Geometry check sheet. Reference: drawing and pictorial views, mm from the part's lowest x, y, z. A direction names the side the tool comes from. Coordinates: 2 decimals unless noted, no trailing zeros. Write each loop counter-clockwise with the first axis right and the second up, starting at its lowest first coordinate (ties: lowest second). Pieces come first, ordered by that corner, then holes. Notation, with made-up numbers: (52, 30.25) - (81, 30.25) arc R36 cw to (81, 69.25) - close; hole circle Ø4 at (3.5, 62). An arc over 180 degrees is marked (long way). Answer as a JSON object with one key per item and string values. Group by question number.
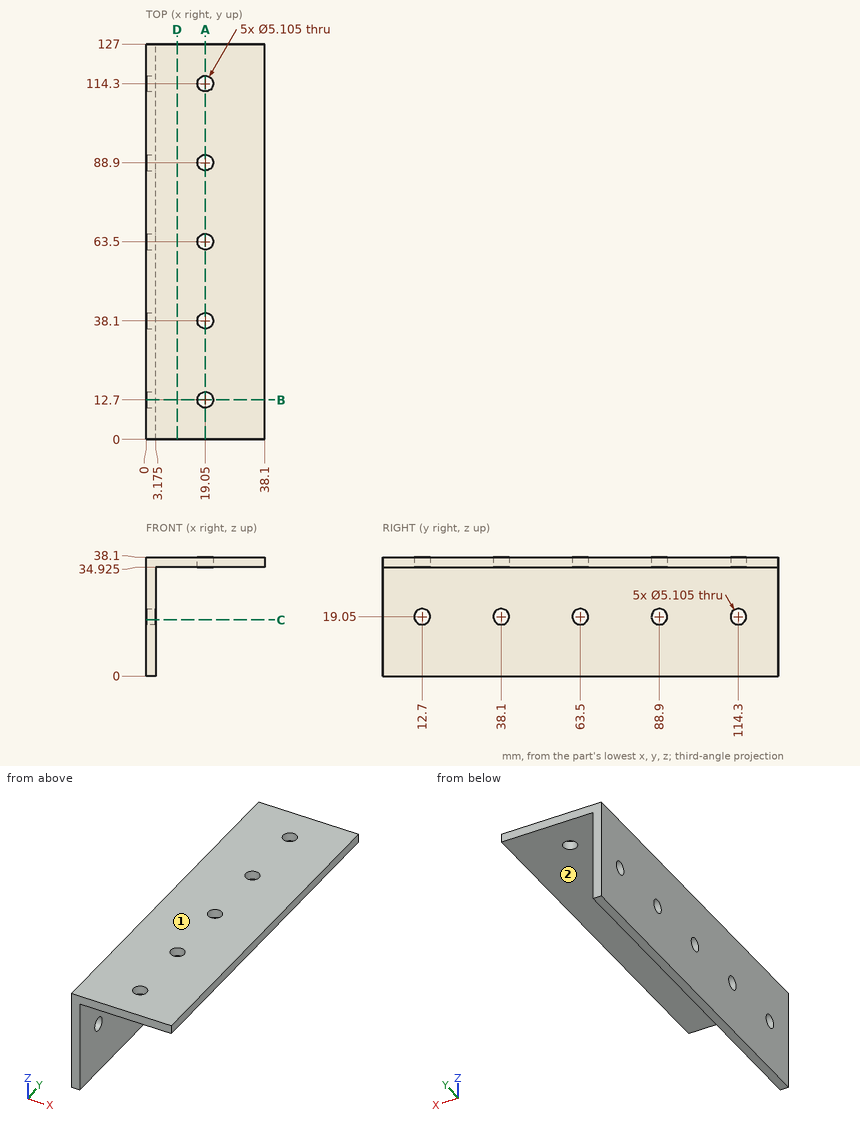
(1) Material ranges on L1, parallel to Y at x = 19.05, z = 37.45; L2, parallel to X at y = 88.9, z = 36.8; L3, parallel to X at y = 33.5, z = 22 (1 decimal), recorded low to high. Write a range as [from, to].
(2) Gauge pin test, flat ends, axial feed: pin 1 (2 mm diameter, centred on x = 31.5, y = 105.5, fed in from -Z) (3 decimals); pin 2 (4 mm diameter, centred on x = 19.05, y = 88.9, fed in from -Z); pin 3 (2 mm diameter, centred on y = 41, z = 30, fed in from +X) (3 decimals). Record the tip position at first contact, or that the pin passes through.
(3) Section check A-A (x = 19.05). Record the cut outline in (y, z) (1 decimal), and give its area (3 significant figures).
(4) Section check D-D (x = 10). Record the cut outline in (y, z) (1 decimal), and give its area (3 significant figures).
(5) Section check C-C (z = 18). Record the cut outline in (x, y) (1 decimal).
(6) Section check B-B (y = 12.7). Record the cut outline in (x, z) (1 decimal).
(7) Set-up check for the marked faces 1 and 2: record each of +Z, -Z, +X, -X, +Y, -Y from which the full face is reachable in a straight line by a thin tool's end or side.
Conclusion:
{
 "1": {"L1": "y = [0, 10.15], [15.25, 35.55], [40.65, 60.95], [66.05, 86.35], [91.45, 111.75], [116.85, 127]", "L2": "x = [0, 16.5], [21.6, 38.1]", "L3": "x = [0, 3.2]"},
 "2": {"pin 1": "stops at z = 34.925", "pin 2": "passes through", "pin 3": "stops at x = 3.175"},
 "3": {"outline": "(0, 34.9) - (10.1, 34.9) - (10.1, 38.1) - (0, 38.1) - close; (15.3, 34.9) - (35.5, 34.9) - (35.5, 38.1) - (15.3, 38.1) - close; (40.7, 34.9) - (60.9, 34.9) - (60.9, 38.1) - (40.7, 38.1) - close; (66.1, 34.9) - (86.3, 34.9) - (86.3, 38.1) - (66.1, 38.1) - close; (91.5, 34.9) - (111.7, 34.9) - (111.7, 38.1) - (91.5, 38.1) - close; (116.9, 34.9) - (127, 34.9) - (127, 38.1) - (116.9, 38.1) - close", "area": "322 mm^2"},
 "4": {"outline": "(0, 34.9) - (127, 34.9) - (127, 38.1) - (0, 38.1) - close", "area": "403 mm^2"},
 "5": {"outline": "(0, 0) - (3.2, 0) - (3.2, 10.4) - (0, 10.4) - close; (0, 15) - (3.2, 15) - (3.2, 35.8) - (0, 35.8) - close; (0, 40.4) - (3.2, 40.4) - (3.2, 61.2) - (0, 61.2) - close; (0, 65.8) - (3.2, 65.8) - (3.2, 86.6) - (0, 86.6) - close; (0, 91.2) - (3.2, 91.2) - (3.2, 112) - (0, 112) - close; (0, 116.6) - (3.2, 116.6) - (3.2, 127) - (0, 127) - close"},
 "6": {"outline": "(0, 0) - (3.2, 0) - (3.2, 16.5) - (0, 16.5) - close; (0, 21.6) - (3.2, 21.6) - (3.2, 34.9) - (16.5, 34.9) - (16.5, 38.1) - (0, 38.1) - close; (21.6, 34.9) - (38.1, 34.9) - (38.1, 38.1) - (21.6, 38.1) - close"},
 "7": {"face 1": "+Z, +X, -X, +Y, -Y", "face 2": "-Z, +X, +Y, -Y"}
}
